For this review, use the dimensioned drawing (mm, ordinates from the lowest corner) and the shaded views. A direction names the side the tool comes from. Give positions to 0.01 mm unless a question says otherwise; leave off trailing zeros. Loops run counter-clockwise (first coordinate to the right, second up) from the corner with the lowest first, then second, coordinate; pieces in that order, holes last. Notation, with made-up numbers: M 19.5,-9 L 53.5,-9 A10 ccw 53.5,3 Z; hole C -5.5,31 d11. An arc over 180 degrees is marked long. Return JSON: item names as keys, results as strings.
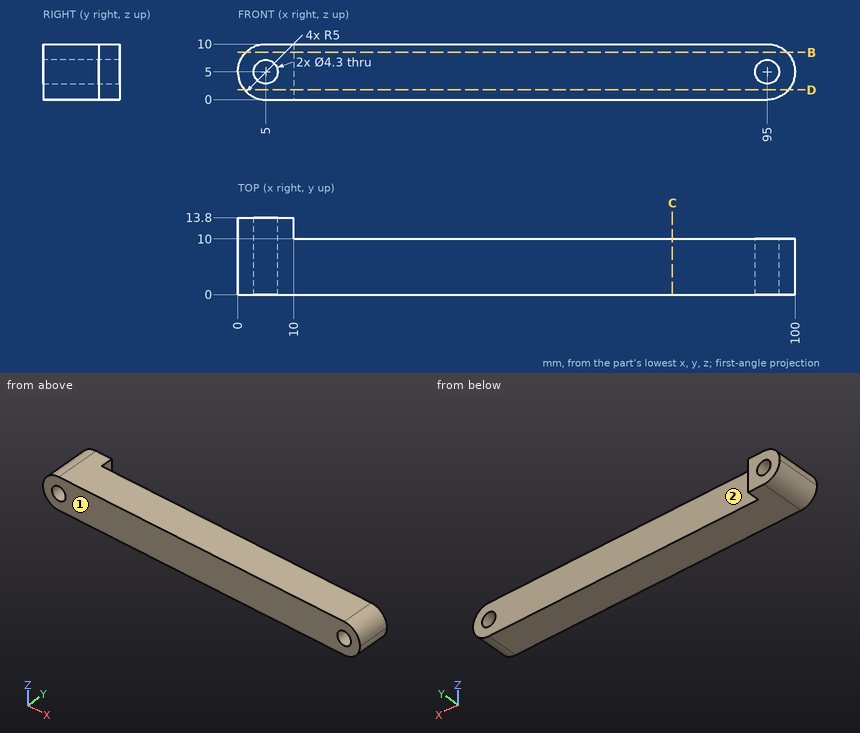
1) Consider section B-B on z = 8.5. Write out the cut boundary in (x, y), then the cut area to 3 significant figures.
From the geometry:
{"outline": "M 1.43,0 L 98.57,0 L 98.57,10 L 10,10 L 10,13.8 L 1.43,13.8 Z", "area": "1,000 mm²"}
2) Tool access review of the marked faces 1 and 2: name each direction out of +Z, -Z, +X, -X, +Y, -Y from which nothing blocks a thin tool from reaching the whole face with its end or side.
From the geometry:
{"face 1": "+Z, -Z, +X, -X, -Y", "face 2": "+Z, -Z, +X, +Y"}
3) Wall thickness on L1, parallel to X at y = 3.75, z = 5; L2, parallel to X at y = 2, z = 4; L3, parallel to Y at x = 11.5, z = 4: over which ranges is each line inside the solid? List them lowest first. Write a range as from..to.
From the geometry:
{"L1": "0..2.85, 7.15..92.85, 97.15..100", "L2": "0.1..3.1, 6.9..93.1, 96.9..99.9", "L3": "0..10"}
4) Consider section C-C on x = 78. Write out the cut boundary in (y, z), then the cut area to 3 significant figures.
From the geometry:
{"outline": "M 0,0 L 10,0 L 10,10 L 0,10 Z", "area": "100 mm²"}
5) Consider section D-D on z = 1.75. Write out the cut boundary in (x, y), then the cut area to 3 significant figures.
From the geometry:
{"outline": "M 1.2,0 L 98.8,0 L 98.8,10 L 10,10 L 10,13.8 L 1.2,13.8 Z", "area": "1,010 mm²"}
6) Insertion check: pin 1 (2 mm diameter, centred on x = 86, z = 9, fed in from +Y); pin 2 (1 mm diameter, centred on y = 3, z = 3.5, fed in from +X); pin 3 (1.9 mm diameter, centred on y = 12.5, z = 4.5, fed in from +X). Each pin has a flat end and moves straight along its axis. Give the tip position at first contact, or say it passes through.
From the geometry:
{"pin 1": "y = 10", "pin 2": "x = 99.9", "pin 3": "x = 10"}
